Autodesk Inventor part; units mm, degrees
ref_plane "YZ Plane" through (0, 0, 0) normal (1, 0, 0) x (0, 1, 0)
ref_plane "XZ Plane" through (0, 0, 0) normal (0, 1, 0) x (-1, 0, 0)
ref_plane "XY Plane" through (0, 0, 0) normal (0, 0, 1) x (1, 0, 0)
sketch "Sketch1" plane through (0, 0, 0) normal (1, 0, 0) x (0, 1, 0)
  line L0 (0, 0) -> (25.4, 0)
  line L1 (25.4, 0) -> (25.4, -25.4)
  line L2 (25.4, -25.4) -> (0, -25.4)
  line L3 (0, -25.4) -> (0, 0)
  line L4 (23.8125, -1.5875) -> (1.5875, -1.5875)
  line L5 (1.5875, -1.5875) -> (1.5875, -23.8125)
  line L6 (1.5875, -23.8125) -> (23.8125, -23.8125)
  line L7 (23.8125, -23.8125) -> (23.8125, -1.5875)
  dimension "d0" = 25.4
  dimension "d1" = 25.4
  dimension "d2" = 1.5875
extrude "Extrusion1" add sketch "Sketch1" along normal mid plane 736.6
chamfer "Chamfer1" distance 25.4 angle 45 2 edges at (-368.3, 12.7, 0) (368.3, 12.7, 0)
properties part number "FRA_TopSide_004" material "Aluminum 6061"
Geometry: final body of the model. Coordinates: model frame, mm. A direction names the side the tool comes from. Round coordinates to 2 decimals unless told otherwise and drop trailing zeros. Loops run counter-clockwise (first coordinate to the right, second up) from the corner with the lowest first, then second, coordinate; pieces in that order, holes last. Notation, with made-up numbers: (-25.5, -23.75) - (-5.5, -23.75) arc R26 ccw to (-5.5, 4.25) - close; hole circle Ø11 at (34.5, -15). An arc over 180 degrees is marked (long way). Write each question's results on one line, items separated by ' | '. Start each with the question number.
1) Mould query, pull axis Z, two halves, no side actions, for faces 1 (the face through (-5, 13, -23.812)), 2 (the face through (355.5, 1.4, -12.6)), 3 (the face through (-5, 13, -25.4)), 4 (the face through (-5, 25.4, -13)). Classes: released by +Z, released by -Z, zero draft, split by the parting line, or undercut.
2) Access query for faces 5 (the face through (-5, 13, -1.588)), 6 (the face through (-5, 13, 0)). Directions: +Z, -Z, +X, -X, +Y, -Y. A direction counts if a zero-diameter tool reaches every point of the face in a straight line with its end or side. Return the directions, or none.
3) Line query: probe 1 along Y at (x, z) = (94.5, -12.5); probe 2 along Z at (x, y) = (-300, 12.5); probe 3 along X at (y, z) = (24.25, -7). Output: solid intervals per line, ascending. Write a range as [from, to].
4) Cut plane B-B on x = -281. Return loops of the section in (y, z).
5) Cut plane C-C on y = 16.5. Return loops of the section in (x, z).
6) First-contact query: P1, Ø12, axis at x = -193, z = -3, coming from the -Y side; P2, Ø1.5, axis at y = 20, z = -4, coming from the +X side. Flat tips, straight axial feed; report the tip coordinate or a pass-through.
7) Cut plane A-A on z = -7. Return loops of the section in (x, y), then the cut area to 3 significant figures.
Verdict:
1) face 1: undercut | face 2: released by +Z | face 3: released by -Z | face 4: zero draft
2) face 5: +X, -X | face 6: +Z, +X, -X, +Y, -Y
3) probe 1: y = [0, 1.59], [23.81, 25.4] | probe 2: z = [-25.4, -23.81], [-1.59, 0] | probe 3: x = [-349.9, 349.9]
4) outline: (0, -25.4) - (25.4, -25.4) - (25.4, 0) - (0, 0) - close; hole (1.59, -23.81) - (23.81, -23.81) - (23.81, -1.59) - (1.59, -1.59) - close
5) outline: (-368.3, -25.4) - (368.3, -25.4) - (366.71, -23.81) - (-366.71, -23.81) - close; (-344.49, -1.59) - (344.49, -1.59) - (342.9, 0) - (-342.9, 0) - close
6) P1: stops at y = 0 | P2: passes through
7) outline: (-349.9, 0) - (349.9, 0) - (349.9, 1.59) - (-349.9, 1.59) - close; (-349.9, 23.81) - (349.9, 23.81) - (349.9, 25.4) - (-349.9, 25.4) - close | area: 2,220 mm2
